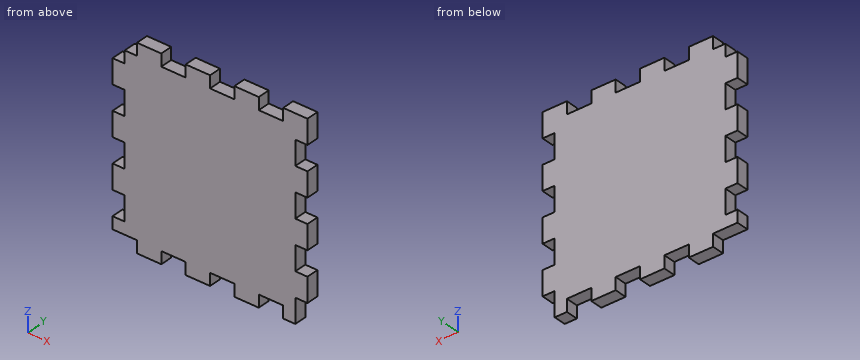
```python
from build123d import *

# Parameters (mm, degrees)
SKETCH1_W           = 101.6
SKETCH1_H           = 101.6
BOSS_EXTRUDE1_DEPTH = 6.35
SKETCH2_W           = 6.35
SKETCH2_H           = 12.7
SKETCH2_H_2         = 6.35
CUT_EXTRUDE1_DEPTH  = 6.35
SKETCH2_3_W         = 6.35
SKETCH2_3_H         = 6.35
SKETCH2_3_W_2       = 12.7
CUT_EXTRUDE2_DEPTH  = 6.35


with BuildPart() as part:
    # Sketch1 → Boss-Extrude1 (new body)
    with BuildSketch(Plane(origin=(0, 0, 0), x_dir=(1, 0, 0), z_dir=(0, 1, 0))):
        with Locations((50.8, 50.8)):
            Rectangle(SKETCH1_W, SKETCH1_H)
    extrude(amount=BOSS_EXTRUDE1_DEPTH)

    # Sketch2 → Cut-Extrude1 (cut)
    with BuildSketch(Plane(origin=(0, 6.35, 0), x_dir=(1, 0, 0), z_dir=(0, 1, 0))):
        with Locations((3.175, 82.55)):
            Rectangle(SKETCH2_W, SKETCH2_H)
        with Locations((3.175, 57.15)):
            Rectangle(SKETCH2_W, SKETCH2_H)
        with Locations((3.175, 31.75)):
            Rectangle(SKETCH2_W, SKETCH2_H)
        with Locations((3.175, 9.525)):
            Rectangle(SKETCH2_W, SKETCH2_H_2)
        with Locations((98.425, 95.25)):
            Rectangle(SKETCH2_W, SKETCH2_H)
        with Locations((98.425, 69.85)):
            Rectangle(SKETCH2_W, SKETCH2_H)
        with Locations((98.425, 44.45)):
            Rectangle(SKETCH2_W, SKETCH2_H)
        with Locations((98.425, 19.05)):
            Rectangle(SKETCH2_W, SKETCH2_H)
    extrude(amount=-CUT_EXTRUDE1_DEPTH, mode=Mode.SUBTRACT)

    # Sketch2_3 → Cut-Extrude2 (cut)
    with BuildSketch(Plane(origin=(0, 6.35, 0), x_dir=(1, 0, 0), z_dir=(0, 1, 0))):
        with Locations((9.525, 98.425)):
            Rectangle(SKETCH2_3_W, SKETCH2_3_H)
        with Locations((31.75, 98.425)):
            Rectangle(SKETCH2_3_W_2, SKETCH2_3_H)
        with Locations((57.15, 98.425)):
            Rectangle(SKETCH2_3_W_2, SKETCH2_3_H)
        with Locations((82.55, 98.425)):
            Rectangle(SKETCH2_3_W_2, SKETCH2_3_H)
        with Locations((82.55, 3.175)):
            Rectangle(SKETCH2_3_W_2, SKETCH2_3_H)
        with Locations((57.15, 3.175)):
            Rectangle(SKETCH2_3_W_2, SKETCH2_3_H)
        with Locations((31.75, 3.175)):
            Rectangle(SKETCH2_3_W_2, SKETCH2_3_H)
        with Locations((9.525, 3.175)):
            Rectangle(SKETCH2_3_W, SKETCH2_3_H)
        with Locations((3.175, 3.175)):
            Rectangle(SKETCH2_3_W, SKETCH2_3_H)
    cut_extrude2 = extrude(amount=-CUT_EXTRUDE2_DEPTH, mode=Mode.SUBTRACT)

    # Mirror2: Cut-Extrude2 across plane
    add(cut_extrude2.mirror(Plane(origin=(0, 0, -50.8), x_dir=(1, 0, 0), z_dir=(0, 0, -1))), mode=Mode.SUBTRACT)


solid = part.part
```
Design review of the part built by this model. Coordinates are the model's own, in mm. Coordinates: 2 decimals unless noted, no trailing zeros. Loops run counter-clockwise (first coordinate to the right, second up) from the corner with the lowest first, then second, coordinate; pieces in that order, holes last. Notation, with made-up numbers: M 53.25,-40 L 91.25,-40 A21 ccw 91.25,-34 Z; hole C 45,22.5 d11. An arc over 180 degrees is marked long. One line per question, with ' | ' between items.
(1) We need section A-A (z = -69). Give the boundary of the cut face in (x, y), and give its area (3 significant figures).
Filled in:
outline: M 0,0 L 95.25,0 L 95.25,6.35 L 0,6.35 Z | area: 605 mm^2
(2) We need section B-B (x = 86.5). Give the boundary of the cut face in (y, z).
Filled in:
outline: M 0,-95.25 L 6.35,-95.25 L 6.35,-6.35 L 0,-6.35 Z
(3) Wall thickness on probe 1 along X at (y, z) = (2.5, -88); probe 2 along Z at (x, y) = (26, 0.75); probe 3 along X at (y, z) = (1, -66.5): over which ranges is each line inside the solid? List them lowest first.
Filled in:
probe 1: x = 6.35 to 101.6 | probe 2: z = -95.25 to -6.35 | probe 3: x = 0 to 95.25
(4) For pin 1 Ø3 at (y, z) = (3, -11) entering from -X; pin 2 Ø1.9 at (x, y) = (58, 2) entering from -Z; pin 3 Ø1.9 at (y, z) = (3, -98.5) entering from -X, all flat-tipped, find the tip position at first contact; note any pin that passes through.
Filled in:
pin 1: stops at x = 6.35 | pin 2: stops at z = -95.25 | pin 3: stops at x = 12.7
